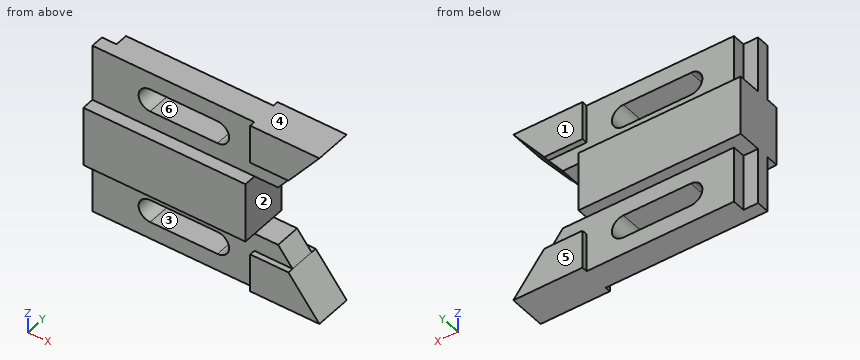
from build123d import *

# Parameters (mm, degrees)
F1_DEPTH = 22.098
F4_DEPTH = 5.842
F5_DEPTH = 8.382
F3_W     = 6.592599522
F3_H     = 25.6785105251
F6_DEPTH = 5.842
F7_DEPTH = 5.842


with BuildPart() as f1:
    # F0 (on Front) → F1 (new body)
    with BuildSketch(Plane.XZ):
        Polygon((-38.0060652603, 0), (35.3999347397, 0), (35.3999347397, 27.1923393011), (-38.0060652603, 27.1923393011), (-38.0060652603, 18.1223209947), (-38.0060652603, 10.0105842575), align=None)
    extrude(amount=F1_DEPTH)

    # F3 (on offset) → F4 (join, symmetric)
    with BuildSketch(Plane.XZ.offset(10.668)):
        Polygon((35.3301167488, 0), (-31.4134657383, 0), (-31.4134657383, -25.6785105251), (35.3301167488, -25.6785105251), (35.3301167488, -8.1525105251), (52.6165383837, -8.1525105251), (46.0923918922, 0), align=None)
        with BuildLine():
            Line((18.6442192644, -17.8938459214), (-11.8596823886, -17.8938459214))
            ThreePointArc((-11.8596823886, -17.8938459214), (-17.0929335328, -12.6605947772), (-11.8596823886, -7.427343633))
            Line((-11.8596823886, -7.427343633), (18.6442192644, -7.427343633))
            ThreePointArc((18.6442192644, -7.427343633), (23.8774704086, -12.6605947772), (18.6442192644, -17.8938459214))
        make_face(mode=Mode.SUBTRACT)
        Polygon((-31.4134657383, 52.8708498262), (-31.4134657383, 27.1923393011), (46.0923918922, 27.1923393011), (52.6165383837, 35.3448498262), (35.3301167488, 35.3448498262), (35.3301167488, 52.8708498262), align=None)
        with BuildLine():
            ThreePointArc((18.6442192644, 45.0756415895), (23.8774704086, 39.8423904453), (18.6442192644, 34.6091393011))
            Line((18.6442192644, 34.6091393011), (-11.8596823886, 34.6091393011))
            ThreePointArc((-11.8596823886, 34.6091393011), (-17.0929335328, 39.8423904453), (-11.8596823886, 45.0756415895))
            Line((-11.8596823886, 45.0756415895), (18.6442192644, 45.0756415895))
        make_face(mode=Mode.SUBTRACT)
    extrude(amount=F4_DEPTH, both=True)

    # F3 (on offset) → F5 (join, symmetric)
    with BuildSketch(Plane.XZ.offset(10.668)):
        Polygon((35.3301167488, -8.1525105251), (35.3301167488, -25.6785105251), (66.6419347397, -25.6785105251), (52.6165383837, -8.1525105251), align=None)
        Polygon((35.3301167488, 35.3448498262), (52.6165383837, 35.3448498262), (66.6419347397, 52.8708498262), (35.3301167488, 52.8708498262), align=None)
    extrude(amount=F5_DEPTH, both=True)

    # F3 (on offset) → F6 (join, through all)
    with BuildSketch(Plane.XZ.offset(10.668)):
        with Locations((-34.7097654993, -12.8392552625)):
            Rectangle(F3_W, F3_H)
    extrude(amount=F6_DEPTH)

    # F3 (on offset) → F7 (join, through all)
    with BuildSketch(Plane.XZ.offset(10.668)):
        with Locations((-34.7097654993, 40.0315945636)):
            Rectangle(F3_W, F3_H)
    extrude(amount=F7_DEPTH)


solid = f1.part
Geometry check sheet. Reference: the model listing, model coordinates, mm. Face numbers are marked on the shaded views. A direction names the side the tool comes from. Coordinates: 2 decimals unless noted, no trailing zeros. Order: outer loops, then holes, each group sorted by start corner. A loop starts at its lowest first (then second) coordinate and runs counter-clockwise, first axis right, second up. Notation, with made-up numbers: (-21.5, -20) -> (-10.5, -20) arc R26 ccw to (-10.5, 11) -> close; hole circle Ø4 at (-6, 80.5). An arc over 180 degrees is marked (long way). Use a Markdown table: item, result. Add a question column.
1. Cross-section at D-D (z = -9.5). Enter the section's corners in (x, y).
2. Material ranges on L1, parallel to Z at x = 4.5, y = -8.5; L2, parallel to Z at x = 45, y = -7.5; L3, parallel to Z at x = -4, y = -1.5, recorded low to high.
3. Cross-section at A-A (x = -0.5). Enter the section's corners in (y, z).
4. Go/stop test with flat-tipped pins: pin 1 Ø11 at (y, z) = (-9.5, 13.5) entering from +X; pin 2 Ø3.5 at (x, z) = (-34, 45) entering from +Y; pin 3 Ø6 at (x, z) = (8, 21.5) entering from +Y; pin 4 Ø13 at (x, z) = (-8, -18) entering from +Y. Record where each tip stops, or that it passes through.
5. Mould release check, pull along Z, two halves, no side actions. Record for the marked faces 4, 5 and 6: pulls with the +Z half, pulls with the -Z half, needs draft (parallel to the pull), parting line crosses it, or undercut.
6. Cross-section at C-C (x = 39.5). Enter the section's corners in (y, z).
7. Set-up check for the marked faces 1, 2 and 3: record each of +Z, -Z, +X, -X, +Y, -Y from which the full face is reachable in a straight line by a thin tool's end or side.
8. Cross-section at B-B (y = -12.5). Enter the section's corners in (x, z), and give its area (3 significant figures).
Filled sheet:
| question | item | result |
|---|---|---|
| 1 | outline | (-38.01, -16.51) -> (-16.03, -16.51) -> (-16.03, -4.83) -> (-31.41, -4.83) -> (-31.41, -10.67) -> (-38.01, -10.67) -> close; (22.82, -16.51) -> (35.33, -16.51) -> (35.33, -19.05) -> (53.69, -19.05) -> (53.69, -2.29) -> (35.33, -2.29) -> (35.33, -4.83) -> (22.82, -4.83) -> close |
| 2 | L1 | -25.68 to -17.89, -7.43 to 34.61, 45.08 to 52.87 |
| 2 | L2 | -25.68 to 0, 27.19 to 52.87 |
| 2 | L3 | 0 to 27.19 |
| 3 | outline | (-22.1, 0) -> (-16.51, 0) -> (-16.51, -7.43) -> (-4.83, -7.43) -> (-4.83, 0) -> (0, 0) -> (0, 27.19) -> (-4.83, 27.19) -> (-4.83, 34.61) -> (-16.51, 34.61) -> (-16.51, 27.19) -> (-22.1, 27.19) -> close; (-16.51, -25.68) -> (-4.83, -25.68) -> (-4.83, -17.89) -> (-16.51, -17.89) -> close; (-16.51, 45.08) -> (-4.83, 45.08) -> (-4.83, 52.87) -> (-16.51, 52.87) -> close |
| 4 | pin 1 | x = 35.4 |
| 4 | pin 2 | y = -10.67 |
| 4 | pin 3 | y = 0 |
| 4 | pin 4 | y = -4.83 |
| 5 | face 4 | pulls with the +Z half |
| 5 | face 5 | needs draft |
| 5 | face 6 | undercut |
| 6 | outline | (-19.05, -25.68) -> (-2.29, -25.68) -> (-2.29, -8.15) -> (-4.83, -8.15) -> (-4.83, 0) -> (-16.51, 0) -> (-16.51, -8.15) -> (-19.05, -8.15) -> close; (-19.05, 35.34) -> (-16.51, 35.34) -> (-16.51, 27.19) -> (-4.83, 27.19) -> (-4.83, 35.34) -> (-2.29, 35.34) -> (-2.29, 52.87) -> (-19.05, 52.87) -> close |
| 7 | face 1 | +Z, -Z, +X, -X, +Y |
| 7 | face 2 | +X, +Y, -Y |
| 7 | face 3 | +Y, -Y |
| 8 | outline | (-38.01, -25.68) -> (66.64, -25.68) -> (46.09, 0) -> (35.4, 0) -> (35.4, 27.19) -> (46.09, 27.19) -> (66.64, 52.87) -> (-38.01, 52.87) -> close; hole (-11.86, -17.89) -> (18.64, -17.89) arc R5.23 ccw to (18.64, -7.43) -> (-11.86, -7.43) arc R5.23 ccw to start; hole (-11.86, 34.61) -> (18.64, 34.61) arc R5.23 ccw to (18.64, 45.08) -> (-11.86, 45.08) arc R5.23 ccw to start |
| 8 | area | 6,030 mm2 |
